Input: part model. Units: mm. Frame: model coordinates. Face numbers are marked on the shaded views. Round coordinates to 2 decimals unless told otherwise and drop trailing zeros. Loops run counter-clockwise (first coordinate to the right, second up) from the corner with the lowest first, then second, coordinate; pieces in that order, holes last. Notation, with made-up numbers: (79.25, 89.25) - (111.25, 89.25) arc R17 cw to (111.25, 111.25) - close; hole circle Ø8 at (25, 39). An arc over 180 degrees is marked (long way). Use CSV: the item, a comma, the result in double quotes. Start each with the question number.
1. Cut plane A-A (y = -14). Return loops of the section in (x, z).
2. Material intervals for probe 1 along Y at (x, z) = (43, 21); probe 2 along X at (y, z) = (39.5, 42.5); probe 3 along X at (y, z) = (41.5, 17.5), sorted ascending. Write a range as from..to.
3. Cut plane D-D (z = 48). Return loops of the section in (x, y), and give its area (3 significant figures).
4. Cut plane C-C (y = 0). Return loops of the section in (x, z), and give its area (3 significant figures).
5. Cut plane B-B (x = 33.5). Return loops of the section in (y, z).
6. Pull-direction query (X, two-part tool) for the marked faces 1, 2, 3 and 4; classes: +X half, -X half, draft (parallel to the pull), parting line (faces both ways), or undercut.
7. Pin query (flat end, axial travel): P1, Ø12, axis at y = -26, z = 12.5, coming from the +X side; P2, Ø10, axis at x = -33, z = 63, coming from the -Y side; P3, Ø3, axis at y = 37.5, z = 67, coming from the +X side. Return the tip coordinate at first contact, or that it passes through.
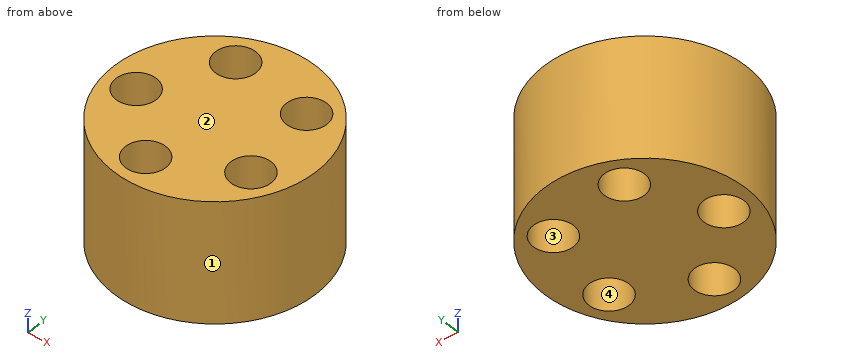
```python
from build123d import *

# Parameters (mm, degrees)
F0_R     = 63.5
F1_DEPTH = 76.2
F2_R     = 12.7
F3_DEPTH = 76.201


with BuildPart() as f1:
    # F0 (on Top) → F1 (new body)
    with BuildSketch(Plane.XY):
        Circle(F0_R)
    extrude(amount=F1_DEPTH)

    # F2 (on face) → F3 (cut, through all)
    with BuildSketch(Plane.XY.offset(76.2)):
        with Locations((-19.843639245, 39.7747719229)):
            Circle(F2_R)
        with Locations((31.6960342644, 31.1635028825)):
            Circle(F2_R)
        with Locations((39.432865729, -20.514667933)):
            Circle(F2_R)
        with Locations((-7.3251829701, -43.842264933)):
            Circle(F2_R)
        with Locations((-43.9600777783, -6.5813419394)):
            Circle(F2_R)
    extrude(amount=-F3_DEPTH, mode=Mode.SUBTRACT)


solid = f1.part
```
Established:
1,outline,"(-61.94, 0) - (-54.27, 0) - (-54.27, 76.2) - (-61.94, 76.2) - close; (-33.65, 0) - (28.53, 0) - (28.53, 76.2) - (-33.65, 76.2) - close; (50.33, 0) - (61.94, 0) - (61.94, 76.2) - (50.33, 76.2) - close"
2,probe 1,"y = -46.73..-32.7, -8.33..25.37, 36.95..46.73"
2,probe 2,"x = -49.72..-32.54, -7.15..22.12, 41.28..49.72"
2,probe 3,"x = -48.06..-32.43, -7.26..24.32, 39.07..48.06"
3,outline,"circle Ø127 at (0, 0); hole circle Ø25.4 at (-43.96, -6.58); hole circle Ø25.4 at (-19.84, 39.77); hole circle Ø25.4 at (-7.33, -43.84); hole circle Ø25.4 at (31.7, 31.16); hole circle Ø25.4 at (39.43, -20.51)"
3,area,"10,100 mm2"
4,outline,"(-63.5, 0) - (-54.82, 0) - (-54.82, 76.2) - (-63.5, 76.2) - close; (-33.1, 0) - (63.5, 0) - (63.5, 76.2) - (-33.1, 76.2) - close"
4,area,"8,020 mm2"
5,outline,"(-53.94, 0) - (-31.74, 0) - (-31.74, 76.2) - (-53.94, 76.2) - close; (-9.29, 0) - (18.59, 0) - (18.59, 76.2) - (-9.29, 76.2) - close; (43.73, 0) - (53.94, 0) - (53.94, 76.2) - (43.73, 76.2) - close"
6,face 1,"parting line"
6,face 2,"draft"
6,face 3,"undercut"
6,face 4,"undercut"
7,P1,"stops at x = 60.27"
7,P2,"stops at y = -56.99"
7,P3,"stops at x = 52.31"
